from build123d import *

# Parameters (mm, degrees)
SKETCH1_R             = 30
SKETCH1_R_2           = 17.5
BOSS_EXTRUDE1_DEPTH   = 48
SKETCH1_R_3           = 12.5
SKETCH1_R_4           = 5
BOSS_EXTRUDE1_2_DEPTH = 48
SKETCH2_R             = 30
SKETCH2_R_2           = 12.5
BOSS_EXTRUDE2_DEPTH   = 8


with BuildPart() as part:
    # Sketch1 → Boss-Extrude1 (new, symmetric)
    with BuildSketch(Plane.XY):
        with Locations((-65, 0)):
            Circle(SKETCH1_R)
        with Locations((-65, 0)):
            Circle(SKETCH1_R_2, mode=Mode.SUBTRACT)
    extrude(amount=BOSS_EXTRUDE1_DEPTH, both=True)



with BuildPart() as body_2:
    # Sketch1 → Boss-Extrude1 2 (new, symmetric)
    with BuildSketch(Plane.XY):
        with Locations((65, 0)):
            Circle(SKETCH1_R_3)
        with Locations((65, 0)):
            Circle(SKETCH1_R_4, mode=Mode.SUBTRACT)
    extrude(amount=BOSS_EXTRUDE1_2_DEPTH, both=True)


with BuildPart() as part_1:
    add(part.part)

    add(body_2.part)  # Boss-Extrude2 merges body 2
    # Sketch2 → Boss-Extrude2 (add)
    with BuildSketch(Plane.XY.offset(33)):
        with BuildLine():
            Line((68.076923077, -19.761896275), (-58.846153846, -39.52379255))
            ThreePointArc((-58.846153846, -39.52379255), (-105, 0), (-58.846153846, 39.52379255))
            Line((-58.846153846, 39.52379255), (68.076923077, 19.761896275))
            ThreePointArc((68.076923077, 19.761896275), (85, 0), (68.076923077, -19.761896275))
        make_face()
        with Locations((-65, 0)):
            Circle(SKETCH2_R, mode=Mode.SUBTRACT)
        with Locations((65, 0)):
            Circle(SKETCH2_R_2, mode=Mode.SUBTRACT)
    boss_extrude2 = extrude(amount=-BOSS_EXTRUDE2_DEPTH)

    # Mirror1: Boss-Extrude2 across plane
    add(boss_extrude2.mirror(Plane.XY))


solid = part_1.part
Verification items for the finished model (mm, model axes). A direction names the side the tool comes from. Give positions to 0.01 mm unless a question says otherwise; leave off trailing zeros. Order: outer loops, then holes, each group sorted by start corner. A loop starts at its lowest first (then second) coordinate and runs counter-clockwise, first axis right, second up. Notation, with made-up numbers: M 78,-22.75 L 85,-22.75 A10 cw 85,-4.75 Z; hole C -11,63 d11. An arc over 180 degrees is marked long. Use one line per item in the form item = value. Start each with the question number.
Q1. Access from +Z, -Z, +X, -X, +Y, -Y to the whole of each face (thin tool, end or side, straight path). Record for faces 1 (the flat face through (-9, 1, 25)), 2 (the cylindrical face through (-94.97, 1.32, -40.39)), 3 (the cylindrical face through (-48.834, -6.703, -0.672)), 4 (the cylindrical face through (55.08, -7.606, 40.605)).
Q2. Section check B-B (z = -27). Enter the section's corners in (x, y).
Q3. Mould release check, pull along X, two halves, no side actions. Record for faces 5 (the flat face through (64.8, -5.4, -48)), 6 (the cylindrical face through (55.08, -7.606, 0.35)), 7 (the cylindrical face through (85, 0, 29)): +X half, -X half, draft (parallel to the pull), parting line (faces both ways), or undercut.
Q4. Go/stop test with flat-tipped pins: pin 1 Ø2 at (x, y) = (30.5, -27.5) entering from +Z; pin 2 Ø24 at (x, y) = (33.5, 8.5) entering from -Z; pin 3 Ø5 at (y, z) = (-9, 29) entering from -X; pin 4 Ø8 at (y, z) = (31.5, 16.5) entering from +X. Record where each tip stops, or that it passes through.
Q5. Section check C-C (y = 0). Count the separate pieces of the cut face and the enclosed holes in it, then the cut area to 3 significant figures.
Q6. Scan lines: line 1 along Y through (x, z) = (65, -12.5); line 2 along Z through (x, y) = (-2, -2.5); line 3 along X through (y, z) = (-8, 13). Record each from-to range of solid material in increasing order. Write a range as [from, to].
Q7. Section check D-D (x = -17.5). Enter the section's corners in (y, z).
Q8. Section check A-A (x = -65). Enter the section's corners in (y, z), then the cut area to 3 significant figures.
Evaluation:
q1.face_1 = none
q1.face_2 = -Z
q1.face_3 = +Z, -Z
q1.face_4 = +Z
q2.outline = M -58.85,-39.52 L 68.08,-19.76 A20 ccw 68.08,19.76 L -58.85,39.52 A40 ccw long Z; hole C -65,0 d35; hole C 65,0 d10
q3.face_5 = draft
q3.face_6 = undercut
q3.face_7 = +X half
q4.pin_1 = through
q4.pin_2 = -33
q4.pin_3 = -104.47
q4.pin_4 = -53.01
q5.separate_pieces = 3
q5.enclosed_holes = 1
q5.area = 5,520 mm2
q6.line_1 = [-12.5, -5], [5, 12.5]
q6.line_2 = [-33, -25], [25, 33]
q6.line_3 = [-93.91, -80.56], [-49.44, -36.09], [55.4, 74.6]
q7.outline = M -33.09,-33 L 33.09,-33 L 33.09,-25 L -33.09,-25 Z; M -33.09,25 L 33.09,25 L 33.09,33 L -33.09,33 Z
q8.outline = M -40,-33 L -30,-33 L -30,-48 L -17.5,-48 L -17.5,48 L -30,48 L -30,33 L -40,33 L -40,25 L -30,25 L -30,-25 L -40,-25 Z; M 17.5,-48 L 30,-48 L 30,-33 L 40,-33 L 40,-25 L 30,-25 L 30,25 L 40,25 L 40,33 L 30,33 L 30,48 L 17.5,48 Z
q8.area = 2,720 mm2
